```python
from build123d import *

# Parameters (mm, degrees)
SKETCH_1_W      = 18.1
SKETCH_1_H      = 16
EXTRUDE_1_DEPTH = 1.66
SKETCH_2_W      = 15.08
SKETCH_2_H      = 16
EXTRUDE_2_DEPTH = 2.18
SKETCH_3_W      = 9.5
SKETCH_3_H      = 9
EXTRUDE_3_DEPTH = 1.96
SKETCH_4_W      = 4.64
SKETCH_4_H      = 16
EXTRUDE_4_DEPTH = 3.6
SKETCH_5_R      = 1.5
EXTRUDE_5_DEPTH = 0.3
CHAMFER_1_SIZE  = 0.3


with BuildPart() as part:
    # 草图1 → 凸台-拉伸1 (new body)
    with BuildSketch(Plane(origin=(0, 0, 0), x_dir=(1, 0, 0), z_dir=(0, 1, 0))):
        with Locations((9.05, 8)):
            Rectangle(SKETCH_1_W, SKETCH_1_H)
    extrude(amount=EXTRUDE_1_DEPTH)

    # 草图2 → 凸台-拉伸2 (add)
    with BuildSketch(Plane.XZ):
        with Locations((8.8, -8)):
            Rectangle(SKETCH_2_W, SKETCH_2_H)
    extrude(amount=EXTRUDE_2_DEPTH)

    # 草图3 → 凸台-拉伸3 (add)
    with BuildSketch(Plane(origin=(0, 1.66, 0), x_dir=(1, 0, 0), z_dir=(0, 1, 0))):
        with Locations((13.35, 8)):
            Rectangle(SKETCH_3_W, SKETCH_3_H)
    extrude(amount=EXTRUDE_3_DEPTH)

    # 草图4 → 凸台-拉伸4 (add)
    with BuildSketch(Plane(origin=(0, 1.66, 0), x_dir=(1, 0, 0), z_dir=(0, 1, 0))):
        with Locations((2.32, 8)):
            Rectangle(SKETCH_4_W, SKETCH_4_H)
    extrude(amount=EXTRUDE_4_DEPTH)

    # 草图5 → 凸台-拉伸5 (add)
    with BuildSketch(Plane.XZ.offset(2.18)):
        with Locations(Location((8.26, -8, 0), (0, 0, 270))):
            Circle(SKETCH_5_R)
    extrude(amount=EXTRUDE_5_DEPTH)

    # 倒角1
    chamfer_1_edges = [part.edges().sort_by_distance(p)[0] for p in [
        (8.26, -2.18, -6.5),
    ]]
    chamfer(chamfer_1_edges, length=CHAMFER_1_SIZE - 0.0001)  # a hair under: the kernel refuses the full size


solid = part.part
```
Design review of the part built by this model. Coordinates are the model's own, in mm. A direction names the side the tool comes from. Coordinates: 2 decimals unless noted, no trailing zeros. Order: outer loops, then holes, each group sorted by start corner. A loop starts at its lowest first (then second) coordinate and runs counter-clockwise, first axis right, second up. Notation, with made-up numbers: (1.25, 72) -> (30.25, 72) arc R26 cw to (30.25, 94) -> close; hole circle Ø6 at (52, 89). An arc over 180 degrees is marked (long way). One line per item, written item: value. Start each with the question number.
Q1. Take a section at C-C, the plane y = -0.5. State the section outline as (x, z) points.
Q2. Mouldability with a two-part tool opening along X and no side actions: class faces 6 (the flat face through (16.34, -1, -8)), 7 (the flat face through (2, 5.26, -8)), 8 (the flat face through (4.64, 3, -8)), 9 (the flat face through (8.6, 3, -8)) as pulls with the +X half, pulls with the -X half, needs draft (parallel to the pull), parting line crosses it, or undercut.
Q3. For probe 1 along X at (y, z) = (3.5, -6); probe 2 along Y at (x, z) = (9.25, -5); probe 3 along Y at (x, z) = (6, -1.75), list the stretches that pass through material, from the lowest coordinate up.
Q4. Insertion check: pin 1 Ø4 at (x, y) = (11.5, 4) entering from +Z; pin 2 Ø1.5 at (y, z) = (-1, -4) entering from +X; pin 3 Ø1 at (x, y) = (13.5, 3) entering from -Z. Each pin has a flat end and moves straight along its axis. Give the tip position at first contact, or say it passes through.
Q5. Tool access review of faces 1 (the flat face through (1.26, -1, -8)), 2 (the flat face through (13, 3, -12.5)), 3 (the flat face through (17, 0, -8)), 4 (the flat face through (13, 3, -3.5)), 5 (the flat face through (13, 3.62, -8)): name each direction out of +Z, -Z, +X, -X, +Y, -Y from which nothing blocks a thin tool from reaching the whole face with its end or side.
Q6. Take a section at A-A, the plane z = -3. State the section outline as (x, y) points, then the cut area to 3 significant figures.
Values follow:
1. outline: (1.26, -16) -> (16.34, -16) -> (16.34, 0) -> (1.26, 0) -> close
2. face 6: pulls with the +X half
2. face 7: needs draft
2. face 8: undercut
2. face 9: undercut
3. probe 1: x = 0 to 4.64, 8.6 to 18.1
3. probe 2: y = -2.18 to 3.62
3. probe 3: y = -2.18 to 1.66
4. pin 1: stops at z = -3.5
4. pin 2: stops at x = 16.34
4. pin 3: stops at z = -12.5
5. face 1: +Z, -Z, -X, -Y
5. face 2: -Z, +X, +Y
5. face 3: +Z, -Z, +X, -Y
5. face 4: +Z, +X, +Y
5. face 5: +Z, -Z, +X, +Y
6. outline: (0, 0) -> (1.26, 0) -> (1.26, -2.18) -> (16.34, -2.18) -> (16.34, 0) -> (18.1, 0) -> (18.1, 1.66) -> (4.64, 1.66) -> (4.64, 5.26) -> (0, 5.26) -> close
6. area: 79.6 mm2
